Build history of the part. All positions in model axes, mm. A direction names the side the tool comes from. Coordinates: 2 decimals unless noted, no trailing zeros. Order: outer loops, then holes, each group sorted by start corner. A loop starts at its lowest first (then second) coordinate and runs counter-clockwise, first axis right, second up. Notation, with made-up numbers: (-26.75, -32.75) - (11.25, -32.75) arc R24 ccw to (11.25, -10.75) - close; hole circle Ø6 at (23.5, 24.25). An arc over 180 degrees is marked (long way). One line per item, written item: value.
from build123d import *

# Parameters (mm, degrees)
SKETCH1_W           = 25.4
SKETCH1_H           = 25.3492
SKETCH1_R           = 4.7625
BOSS_EXTRUDE1_DEPTH = 1.64338
SKETCH2_W           = 25.4
SKETCH2_H           = 1.64338
BOSS_EXTRUDE2_DEPTH = 7.98322
SKETCH3_W           = 5.588
SKETCH3_H           = 1.64338
BOSS_EXTRUDE3_DEPTH = 4.318
SKETCH4_W           = 25.4
SKETCH4_H           = 1.64338
BOSS_EXTRUDE4_DEPTH = 25.50922
CUT_EXTRUDE1_DEPTH  = 1.64338
FILLET1_R           = 1.524
FILLET2_R           = 3.16738


with BuildPart() as part:
    # Sketch1 → Boss-Extrude1 (new body)
    with BuildSketch(Plane(origin=(0, 0, 0), x_dir=(1, 0, 0), z_dir=(0, 1, 0))):
        Rectangle(SKETCH1_W, SKETCH1_H)
        Circle(SKETCH1_R, mode=Mode.SUBTRACT)
    extrude(amount=BOSS_EXTRUDE1_DEPTH)

    # Sketch2 → Boss-Extrude2 (add)
    with BuildSketch(Plane(origin=(0, 1.64338, 0), x_dir=(1, 0, 0), z_dir=(0, 1, 0))):
        with Locations((0, -11.85291)):
            Rectangle(SKETCH2_W, SKETCH2_H)
    extrude(amount=BOSS_EXTRUDE2_DEPTH)

    # Sketch3 → Boss-Extrude3 (add)
    with BuildSketch(Plane(origin=(0, 9.6266, 0), x_dir=(1, 0, 0), z_dir=(0, 1, 0))):
        with Locations((-9.906, -11.85291)):
            Rectangle(SKETCH3_W, SKETCH3_H)
        with Locations((9.906, -11.85291)):
            Rectangle(SKETCH3_W, SKETCH3_H)
    extrude(amount=BOSS_EXTRUDE3_DEPTH)

    # Sketch4 → Boss-Extrude4 (add)
    with BuildSketch(Plane(origin=(0, 1.64338, 0), x_dir=(1, 0, 0), z_dir=(0, 1, 0))):
        with Locations((0, 11.85291)):
            Rectangle(SKETCH4_W, SKETCH4_H)
    extrude(amount=BOSS_EXTRUDE4_DEPTH)

    # Sketch5 → Cut-Extrude1 (cut)
    with BuildSketch(Plane(origin=(0, 0, -12.6746), x_dir=(-1, 0, 0), z_dir=(0, 0, -1))):
        with BuildLine():
            Line((-3.1242, 9.1186), (-3.1242, 18.670657305))
            ThreePointArc((-3.1242, 18.670657305), (0, 24.003), (3.1242, 18.670657305))
            Line((3.1242, 18.670657305), (3.1242, 9.1186))
            Line((3.1242, 9.1186), (1.524, 9.1186))
            Line((1.524, 9.1186), (1.524, 17.180635644))
            ThreePointArc((1.524, 17.180635644), (0, 16.8402), (-1.524, 17.180635644))
            Line((-1.524, 17.180635644), (-1.524, 9.1186))
            Line((-1.524, 9.1186), (-3.1242, 9.1186))
        make_face()
    extrude(amount=-CUT_EXTRUDE1_DEPTH, mode=Mode.SUBTRACT)

    # Fillet1
    fillet1_edges = [part.edges().sort_by_distance(p)[0] for p in [
        (0, 1.64338, 11.03122),
        (0, 1.64338, -11.03122),
    ]]
    fillet(fillet1_edges, radius=FILLET1_R)

    # Fillet2
    fillet2_edges = [part.edges().sort_by_distance(p)[0] for p in [
        (0, 0, -12.6746),
        (0, 0, 12.6746),
    ]]
    fillet(fillet2_edges, radius=FILLET2_R)


solid = part.part
1. Band-saw the part on A-A, the plane z = 0. Give the cut face in (x, y), and give its area (3 significant figures).
Values found:
outline: (-12.7, 0) - (-4.76, 0) - (-4.76, 1.64) - (-12.7, 1.64) - close; (4.76, 0) - (12.7, 0) - (12.7, 1.64) - (4.76, 1.64) - close
area: 26.1 mm2
2. Two-plate mould, pull along Z, no slides. Class faces 6 (the face through (0.18, 0.9, 11.72)), 7 (the face through (10, 13.945, 12)), 8 (the face through (-3.78, 0.81, 2.9)): pulls with the +Z half, pulls with the -Z half, needs draft (parallel to the pull), parting line crosses it, or undercut.
Values found:
face 6: pulls with the +Z half
face 7: needs draft
face 8: undercut
3. Band-saw the part on B-B, the plane y = 11. Give the cut face in (x, z), and give its area (3 significant figures).
Values found:
outline: (-12.7, -12.67) - (-3.12, -12.67) - (-3.12, -11.03) - (-12.7, -11.03) - close; (-12.7, 11.03) - (-7.11, 11.03) - (-7.11, 12.67) - (-12.7, 12.67) - close; (-1.52, -12.67) - (1.52, -12.67) - (1.52, -11.03) - (-1.52, -11.03) - close; (3.12, -12.67) - (12.7, -12.67) - (12.7, -11.03) - (3.12, -11.03) - close; (7.11, 11.03) - (12.7, 11.03) - (12.7, 12.67) - (7.11, 12.67) - close
area: 54.8 mm2
4. Flat gauge pins, fed straight in: P1, Ø0.8, axis at x = -9, z = 11.5, coming from the +Y side; P2, Ø8, axis at x = -4, z = 1.5, coming from the +Y side; P3, Ø12, axis at x = -4, y = 20.5, coming from the +Z side; P4, Ø9.5, axis at x = 0, y = 20.42, coming from the -Z side. Where does each tip first touch, or does it go through?
Values found:
P1: stops at y = 13.94
P2: stops at y = 1.64
P3: stops at z = -11.03
P4: stops at z = -12.67
5. 3-axis set-ups, long thin cutter, end or side, ignore diameter. For faces 1 (the face through (-0.02, 16.84, -11.86)), 2 (the face through (-10, 13.945, 12)), 3 (the face through (7.112, 12, 12)), 4 (the face through (0, 7, 11.031)), 5 (the face through (2, 9.119, -12)): which of +Z, -Z, +X, -X, +Y, -Y reach the whole face in a straight line?
Values found:
face 1: +Z, -Z
face 2: +Z, +X, -X, +Y
face 3: +Z, +Y
face 4: +X, -X, +Y
face 5: -Z
6. Probe line 1 along Z through (x, y) = (9.5, 7.5); line 2 along X through (y, z) = (0.3, 0); line 3 along Y through (x, z) = (7, -6.5). List the from-to ranges inside material, lowest first.
Values found:
line 1: z = -12.67 to -11.03, 11.03 to 12.67
line 2: x = -12.7 to -4.76, 4.76 to 12.7
line 3: y = 0 to 1.64
7. Band-saw the part on D-D, the plane y = 21.75. Give the cut face in (x, z), and give its area (3 significant figures).
Values found:
outline: (-12.7, -12.67) - (-3.33, -12.67) - (-3.33, -11.03) - (-12.7, -11.03) - close; (3.33, -12.67) - (12.7, -12.67) - (12.7, -11.03) - (3.33, -11.03) - close
area: 30.8 mm2
8. Band-saw the part on C-C, the plane x = 0. Give the cut face in (y, z).
Values found:
outline: (0, -9.51) arc R3.17 ccw to (3.17, -12.67) - (16.84, -12.67) - (16.84, -11.03) - (3.17, -11.03) arc R1.52 cw to (1.64, -9.51) - (1.64, -4.76) - (0, -4.76) - close; (0, 4.76) - (1.64, 4.76) - (1.64, 9.51) arc R1.52 cw to (3.17, 11.03) - (9.63, 11.03) - (9.63, 12.67) - (3.17, 12.67) arc R3.17 ccw to (0, 9.51) - close; (24, -12.67) - (27.15, -12.67) - (27.15, -11.03) - (24, -11.03) - close
